Source: CAD feature listing. Evaluate the final solid. Frame: model axes, mm. A direction names the side the tool comes from. Round coordinates to 2 decimals unless told otherwise and drop trailing zeros. Loops run counter-clockwise (first coordinate to the right, second up) from the corner with the lowest first, then second, coordinate; pieces in that order, holes last.
(1) Section D-D, the plane z = 10.5. Return the cut outline in (x, y) (3 decimals).
(2) Section A-A, the plane z = 5. Return the cut outline in (x, y) (3 decimals).
(3) Section B-B, the plane x = 5. Return the cut outline in (y, z) (3 decimals), plus the area to 3 significant figures.
(4) Set-up query: faces 5 (the flat face through (-15, 7.5, 3)), 6 (the flat face through (15, 7.5, 3)), 7 (the flat face through (15, -7.5, 3)), 8 (the flat face through (13.6, 0, 5)). Return all of +Z, -Z, +X, -X, +Y, -Y with unobstructed straight access to the full face (end or side cutting, diameter ignored); none if empty.
(5) First-contact query: pin 1 Ø1.1 at (y, z) = (-9, 1.5) entering from +X; pin 2 Ø6 at (x, z) = (-1.5, 3.5) entering from +Y; pin 3 Ø4 at (y, z) = (-5.5, 3.5) entering from +X; pin 4 Ø0.7 at (y, z) = (8, 2) entering from -X. Flat tips, straight axial feed; report the tip coordinate or a pass-through.
(6) Material intervals for probe 1 along X at (y, z) = (0.25, 3.75); probe 2 along X at (y, z) = (-0.5, 9.5); probe 3 along Z at (x, y) = (0, 9), sorted ascending.
(7) Section C-C, the plane y = 0. Return the cut outline in (x, z) (3 decimals), plus the area to 3 significant figures.
(8) Mould query, pull axis Y, two halves, no side actions, for faces 1 (the cylindrical face through (3.576, 0.063, 7.089)), 2 (the flat face through (0, -9.75, 1)), 3 (the cylindrical face through (-14.5, 0.99, 1.87)), 4 (the cylindrical face through (20.7, -1.26, 1.87)). Classes: pulls with the +Y half, pulls with the -Y half, needs draft (parallel to the pull), parting line crosses it, or undercut.
```python
from build123d import *

# Parameters (mm, degrees)
F1_DEPTH = 6.8
F2_W     = 27.2
F2_H     = 19.5
F3_DEPTH = 4
F4_R     = 3.3
F5_DEPTH = 3.8
F6_R     = 1.425
F7_DEPTH = 8.7


with BuildPart() as f1:
    # F0 (on Top) → F1 (new body)
    with BuildSketch(Plane.XY):
        with BuildLine():
            Line((13.6, 7.5), (13.6, 9.75))
            Line((13.6, 9.75), (-13.6, 9.75))
            Line((-13.6, 9.75), (-13.6, 7.5))
            Line((-13.6, 7.5), (-15.6, 7.5))
            ThreePointArc((-15.6, 7.5), (-21.931769, 0), (-15.6, -7.5))
            Line((-15.6, -7.5), (-13.6, -7.5))
            Line((-13.6, -7.5), (-13.6, -9.75))
            Line((-13.6, -9.75), (13.6, -9.75))
            Line((13.6, -9.75), (13.6, -7.5))
            Line((13.6, -7.5), (15.6, -7.5))
            ThreePointArc((15.6, -7.5), (21.931769, 0), (15.6, 7.5))
            Line((15.6, 7.5), (13.6, 7.5))
        make_face()
    extrude(amount=F1_DEPTH)

    # F2 (on face) → F3 (cut)
    with BuildSketch(Plane.XY.offset(6.8)):
        Rectangle(F2_W, F2_H)
    extrude(amount=-F3_DEPTH, mode=Mode.SUBTRACT)

    # F4 (on Top) → F5 (cut)
    with BuildSketch(Plane.XY):
        with Locations((17.65, 0)):
            Circle(F4_R)
        with Locations((-17.65, 0)):
            Circle(F4_R)
    extrude(amount=F5_DEPTH, mode=Mode.SUBTRACT)

    # F6 (on face) → F7 (join)
    with BuildSketch(Plane.XY.offset(2.8)):
        with Locations((5, 0)):
            Circle(F6_R)
        with Locations((-5, 0)):
            Circle(F6_R)
    extrude(amount=F7_DEPTH)


solid = f1.part
```
Output values:
1. outline: circle Ø2.85 at (-5, 0); circle Ø2.85 at (5, 0)
2. outline: (-15.6, -7.5) - (-13.6, -7.5) - (-13.6, 7.5) - (-15.6, 7.5) arc R7.608 ccw to start; circle Ø2.85 at (-5, 0); circle Ø2.85 at (5, 0); (13.6, -7.5) - (15.6, -7.5) arc R7.608 ccw to (15.6, 7.5) - (13.6, 7.5) - close
3. outline: (-9.75, 0) - (9.75, 0) - (9.75, 2.8) - (1.425, 2.8) - (1.425, 11.5) - (-1.425, 11.5) - (-1.425, 2.8) - (-9.75, 2.8) - close
3. area: 79.4 mm2
4. face 5: +Z, -Z, -X, +Y
4. face 6: +Z, -Z, +X, +Y
4. face 7: +Z, -Z, +X, -Y
4. face 8: +Z, +Y, -Y
5. pin 1: stops at x = 13.6
5. pin 2: stops at y = 9.75
5. pin 3: stops at x = 21.08
5. pin 4: stops at x = -13.6
6. probe 1: x = -21.93 to -20.94, -14.36 to -13.6, -6.4 to -3.6, 3.6 to 6.4, 13.6 to 14.36, 20.94 to 21.93
6. probe 2: x = -6.33 to -3.67, 3.67 to 6.33
6. probe 3: z = 0 to 2.8
7. outline: (-21.932, 0) - (-20.95, 0) - (-20.95, 3.8) - (-14.35, 3.8) - (-14.35, 0) - (14.35, 0) - (14.35, 3.8) - (20.95, 3.8) - (20.95, 0) - (21.932, 0) - (21.932, 6.8) - (13.6, 6.8) - (13.6, 2.8) - (6.425, 2.8) - (6.425, 11.5) - (3.575, 11.5) - (3.575, 2.8) - (-3.575, 2.8) - (-3.575, 11.5) - (-6.425, 11.5) - (-6.425, 2.8) - (-13.6, 2.8) - (-13.6, 6.8) - (-21.932, 6.8) - close
7. area: 189 mm2
8. face 1: parting line crosses it
8. face 2: pulls with the -Y half
8. face 3: undercut
8. face 4: undercut
